```python
from build123d import *
from OCP.BRepFilletAPI import BRepFilletAPI_MakeChamfer

# Parameters (mm, degrees)
SKETCH1_R           = 74.5
SKETCH1_R_2         = 4
SKETCH1_R_3         = 17.5
BOSS_EXTRUDE1_DEPTH = 2.5
CHAMFER1_SIZE       = 0.5
CHAMFER1_SIZE2      = 0.866025404


# Read off the part's stored shape, not the designer's step: CirPattern1
with BuildPart() as part:
    # Sketch1 → Boss-Extrude1 (new, symmetric)
    with BuildSketch(Plane(origin=(0, 0, 0), x_dir=(1, 0, 0), z_dir=(0, 1, 0))):
        with Locations(Location((0, 0, 0), (0, 0, 270))):
            Circle(SKETCH1_R)
        with Locations(Location((0, 50, 0), (0, 0, 270))):
            Circle(SKETCH1_R_2, mode=Mode.SUBTRACT)
        with Locations(Location((35.355339059, 35.355339059, 0), (0, 0, 270))):
            Circle(SKETCH1_R_2, mode=Mode.SUBTRACT)
        with Locations(Location((50, 0, 0), (0, 0, 270))):
            Circle(SKETCH1_R_2, mode=Mode.SUBTRACT)
        with Locations(Location((35.355339059, -35.355339059, 0), (0, 0, 270))):
            Circle(SKETCH1_R_2, mode=Mode.SUBTRACT)
        with Locations(Location((0, -50, 0), (0, 0, 270))):
            Circle(SKETCH1_R_2, mode=Mode.SUBTRACT)
        with Locations(Location((-35.355339059, -35.355339059, 0), (0, 0, 270))):
            Circle(SKETCH1_R_2, mode=Mode.SUBTRACT)
        with Locations(Location((-50, 0, 0), (0, 0, 270))):
            Circle(SKETCH1_R_2, mode=Mode.SUBTRACT)
        with Locations(Location((-35.355339059, 35.355339059, 0), (0, 0, 270))):
            Circle(SKETCH1_R_2, mode=Mode.SUBTRACT)
        with Locations(Location((0, 0, 0), (0, 0, 270))):
            Circle(SKETCH1_R_3, mode=Mode.SUBTRACT)
    extrude(amount=BOSS_EXTRUDE1_DEPTH, both=True)

    # Sketch2 → Revolve1 (revolve)
    with BuildSketch(Plane(origin=(0, 0, 0), x_dir=(0, 0, -1), z_dir=(1, 0, 0)), mode=Mode.PRIVATE) as revolve1_sk:
        Polygon((-62.227241336, 2.5), (-54, 7.25), (-54, -7.25), (-62.227241336, -2.5), align=None)
    revolve(revolve1_sk.sketch.rotate(Axis((0, 2.5, 50), (0, 1, 0)), 180), axis=Axis((0, 2.5, 50), (0, 1, 0)))

    # Chamfer1: one chamfer whose edges measure the first distance from different faces: ONE call of the kernel's chamfer builder (chamfer() names one face for all edges)
    chamfer1_edges_1 = [part.edges().sort_by_distance(p)[0] for p in [
        (0, -2.5, -17.5),
    ]]
    chamfer1_side_1 = [part.faces().sort_by_distance(p)[0] for p in [
        (0, 0, -17.5),
    ]]
    chamfer1_edges_2 = [part.edges().sort_by_distance(p)[0] for p in [
        (0, 2.5, -17.5),
    ]]
    chamfer1_side_2 = [part.faces().sort_by_distance(p)[0] for p in [
        (0, 2.5, -72.392821792),
    ]]
    chamfer1_edges_3 = [part.edges().sort_by_distance(p)[0] for p in [
        (0, -2.5, -74.5),
    ]]
    chamfer1_side_3 = [part.faces().sort_by_distance(p)[0] for p in [
        (0, -2.5, -72.392821792),
    ]]
    chamfer1_edges_4 = [part.edges().sort_by_distance(p)[0] for p in [
        (0, -7.25, 54),
        (0, 7.25, 54),
    ]]
    chamfer1_edges_5 = [part.edges().sort_by_distance(p)[0] for p in [
        (0, 2.5, -74.5),
    ]]
    chamfer1_side_5 = [part.faces().sort_by_distance(p)[0] for p in [
        (0, 0, -74.5),
    ]]
    chamfer1 = BRepFilletAPI_MakeChamfer(part.part.solid().wrapped)
    for e in chamfer1_edges_1:
        chamfer1.Add(CHAMFER1_SIZE, CHAMFER1_SIZE2, e.wrapped, chamfer1_side_1[0].wrapped)  # the first distance lies on this face
    for e in chamfer1_edges_2:
        chamfer1.Add(CHAMFER1_SIZE, CHAMFER1_SIZE2, e.wrapped, chamfer1_side_2[0].wrapped)  # the first distance lies on this face
    for e in chamfer1_edges_3:
        chamfer1.Add(CHAMFER1_SIZE, CHAMFER1_SIZE2, e.wrapped, chamfer1_side_3[0].wrapped)  # the first distance lies on this face
    for e in chamfer1_edges_4:
        chamfer1.Add(CHAMFER1_SIZE, e.wrapped)
    for e in chamfer1_edges_5:
        chamfer1.Add(CHAMFER1_SIZE, CHAMFER1_SIZE2, e.wrapped, chamfer1_side_5[0].wrapped)  # the first distance lies on this face
    add(Compound.cast(chamfer1.Shape()), mode=Mode.REPLACE)

    # CirPattern1 outline → CirPattern1 (revolve)
    with BuildSketch(Plane(origin=(-35.355339059, 0, 35.355339059), x_dir=(1, 0, 0), z_dir=(0, 0, 1))):
        Polygon((4, -6.75), (4.433012702, -7), (12.227241336, -2.5), (4, -2.5), align=None)
        Polygon((4, 2.5), (12.227241336, 2.5), (4.433012702, 7), (4, 6.75), align=None)
    revolve(axis=Axis((-35.355339059, 0, 35.355339059), (0, 1, 0)))

    # CirPattern1 2 outline → CirPattern1 2 (revolve)
    with BuildSketch(Plane(origin=(-50, 0, 0), x_dir=(1, 0, 0), z_dir=(0, 0, 1))):
        Polygon((4, -6.75), (4.433012702, -7), (12.227241336, -2.5), (4, -2.5), align=None)
        Polygon((4, 2.5), (12.227241336, 2.5), (4.433012702, 7), (4, 6.75), align=None)
    revolve(axis=Axis((-50, 0, 0), (0, 1, 0)))

    # CirPattern1 3 outline → CirPattern1 3 (revolve)
    with BuildSketch(Plane(origin=(-35.355339059, 0, -35.355339059), x_dir=(1, 0, 0), z_dir=(0, 0, 1))):
        Polygon((4, -6.75), (4.433012702, -7), (12.227241336, -2.5), (4, -2.5), align=None)
        Polygon((4, 2.5), (12.227241336, 2.5), (4.433012702, 7), (4, 6.75), align=None)
    revolve(axis=Axis((-35.355339059, 0, -35.355339059), (0, 1, 0)))

    # CirPattern1 4 outline → CirPattern1 4 (revolve)
    with BuildSketch(Plane.XY.offset(-50)):
        Polygon((4, -6.75), (4.433012702, -7), (12.227241336, -2.5), (4, -2.5), align=None)
        Polygon((4, 2.5), (12.227241336, 2.5), (4.433012702, 7), (4, 6.75), align=None)
    revolve(axis=Axis((0, 0, -50), (0, 1, 0)))

    # CirPattern1 5 outline → CirPattern1 5 (revolve)
    with BuildSketch(Plane(origin=(35.355339059, 0, -35.355339059), x_dir=(1, 0, 0), z_dir=(0, 0, 1))):
        Polygon((4, -6.75), (4.433012702, -7), (12.227241336, -2.5), (4, -2.5), align=None)
        Polygon((4, 2.5), (12.227241336, 2.5), (4.433012702, 7), (4, 6.75), align=None)
    revolve(axis=Axis((35.355339059, 0, -35.355339059), (0, 1, 0)))

    # CirPattern1 6 outline → CirPattern1 6 (revolve)
    with BuildSketch(Plane(origin=(50, 0, 0), x_dir=(1, 0, 0), z_dir=(0, 0, 1))):
        Polygon((4, -6.75), (4.433012702, -7), (12.227241336, -2.5), (4, -2.5), align=None)
        Polygon((4, 2.5), (12.227241336, 2.5), (4.433012702, 7), (4, 6.75), align=None)
    revolve(axis=Axis((50, 0, 0), (0, 1, 0)))

    # CirPattern1 7 outline → CirPattern1 7 (revolve)
    with BuildSketch(Plane(origin=(35.355339059, 0, 35.355339059), x_dir=(1, 0, 0), z_dir=(0, 0, 1))):
        Polygon((4, -6.75), (4.433012702, -7), (12.227241336, -2.5), (4, -2.5), align=None)
        Polygon((4, 2.5), (12.227241336, 2.5), (4.433012702, 7), (4, 6.75), align=None)
    revolve(axis=Axis((35.355339059, 0, 35.355339059), (0, 1, 0)))


solid = part.part
```
Here's how the part is built. I have some questions about the finished solid (model axes, mm). A direction names the side the tool comes from. Give positions to 0.01 mm unless a question says otherwise; leave off trailing zeros. Answer as a JSON object with one key per item and string values. Group by question number.
Item 1: Which directions (+Z, -Z, +X, -X, +Y, -Y) give clear straight access to the entire face, cutting with the end or side of a thin tool? Please do faces 1 (the flat face through (-15, -2.5, 15)), 2 (the conical face through (-1.04, 6.78, -45.3)).
Item 2: Please list where these lines run through material, in increasing order: probe 1 along X at (y, z) = (-1.2, 0); probe 2 along X at (y, z) = (-3.5, 39); probe 3 along X at (y, z) = (2.25, -34).
Item 3: For P1, Ø3, axis at x = 22.5, y = -3, coming from the -Z side; P2, Ø3, axis at y = 0, z = 31.5, coming from the -X side; P3, Ø3, axis at y = -4.5, z = -39, coming from the -X side, each with a flat end and sliding along its axis, tell me the tip position at first contact or that it passes through.
Result set:
{
 "1": {"face 1": "-Y", "face 2": "+Y"},
 "2": {"probe 1": "-74.5 to -54, -46 to -17.5, 17.5 to 46, 54 to 74.5", "probe 2": "-45.2 to -37, -33.71 to -25.51, 25.51 to 33.71, 37 to 45.2", "probe 3": "-65.8 to -39.12, -31.59 to 31.59, 39.12 to 65.8"},
 "3": {"P1": "z = -71.22", "P2": "x = -68.19", "P3": "x = -46.16"}
}
